from build123d import *

# Parameters (mm, degrees)
BOSS_EXTRUDE1_DEPTH     = 10
CUT_EXTRUDE1_DEPTH      = 26.734218465
CUT_EXTRUDE1_DEPTH_BACK = 26.734218465
SKETCH2_R               = 3.1
SKETCH3_R               = 2
CUT_EXTRUDE2_DEPTH      = 8.5


with BuildPart() as part:
    # Sketch1 → Boss-Extrude1 (new, symmetric)
    with BuildSketch(Plane.XY):
        with BuildLine():
            Line((-8, -21.5), (8, -21.5))
            ThreePointArc((8, -21.5), (9.414213562, -20.914213562), (10, -19.5))
            Line((10, -19.5), (10, -2))
            ThreePointArc((10, -2), (9.414213562, -0.585786438), (8, 0))
            Line((8, 0), (-8, 0))
            ThreePointArc((-8, 0), (-9.414213562, -0.585786438), (-10, -2))
            Line((-10, -2), (-10, -19.5))
            ThreePointArc((-10, -19.5), (-9.414213562, -20.914213562), (-8, -21.5))
        make_face()
    extrude(amount=BOSS_EXTRUDE1_DEPTH, both=True)

    # Sketch2 → Cut-Extrude1 (cut, two sides: drawn at the far end of the back side and taken through both)
    with BuildSketch(Plane(origin=(0, 0, 0), x_dir=(0, 0, -1), z_dir=(1, 0, 0)).offset(-CUT_EXTRUDE1_DEPTH_BACK)):
        with Locations((0, -9.5)):
            Circle(SKETCH2_R)
    extrude(amount=CUT_EXTRUDE1_DEPTH + CUT_EXTRUDE1_DEPTH_BACK, mode=Mode.SUBTRACT)

    # Sketch3 → Cut-Extrude2 (cut)
    with BuildSketch(Plane(origin=(0, -21.5, 0), x_dir=(1, 0, 0), z_dir=(0, 1, 0))):
        with Locations(Location((0, 0, 0), (0, 0, 270))):
            Circle(SKETCH3_R)
    extrude(amount=CUT_EXTRUDE2_DEPTH, mode=Mode.SUBTRACT)


solid = part.part
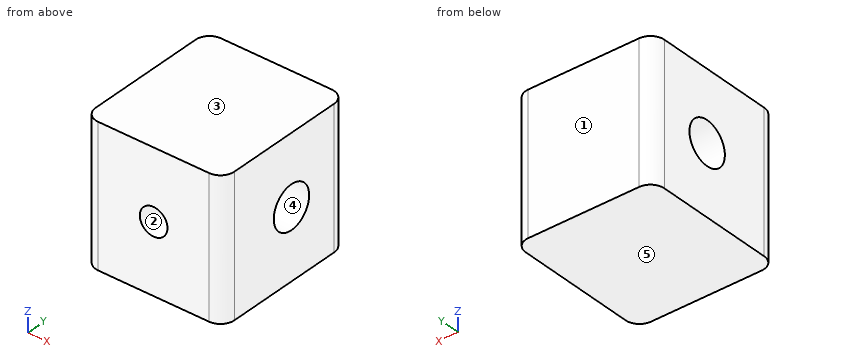
Read the model definition and answer for the solid it produces. Units are mm, in the model's axes. Face numbers are marked on the shaded views. A direction names the side the tool comes from. Round coordinates to 2 decimals unless told otherwise and drop trailing zeros. Loops run counter-clockwise (first coordinate to the right, second up) from the corner with the lowest first, then second, coordinate; pieces in that order, holes last.
Q1. This flat-tipped pin is pushed along its axis until it touches: pin 1 (3.5 mm diameter, centred on x = 0, z = 0, fed in from -Y). Where does it stop, or does it pass through?
Q2. Determine the mould class of the marked faces 3, 4 and 5 for opening direction Z: released by +Z, released by -Z, zero draft, split by the parting line, or undercut.
Q3. Consider probe 1 along Z at (x, y) = (0, -9.5); probe 2 along Y at (x, z) = (-7, 0); probe 3 along X at (y, z) = (-19.5, 0). Determine where each line is inside the solid, lowest interval first.
Q4. Section D-D on y = -18 is taken. Write down the section's boundary in (x, z), and give its area (3 significant figures).
Q5. Which of the six approach directions +Z, -Z, +X, -X, +Y, -Y give full straight-line access (tool end or side, diameter ignored) to the marked faces 1 and 2?
Q6. Section C-C on x = 0 is taken. Write down the section's boundary in (y, z), and give its area (3 significant figures).
Q7. Section A-A on y = -9.5 is taken. Write down the section's boundary in (x, z).
Q8. Section B-B on z = 0 is taken. Write down the section's boundary in (x, y).
Output:
1. pin 1: stops at y = -13
2. face 3: released by +Z
2. face 4: undercut
2. face 5: released by -Z
3. probe 1: z = -10 to -3.1, 3.1 to 10
3. probe 2: y = -21.5 to -12.6, -6.4 to 0
3. probe 3: x = -10 to -2, 2 to 10
4. outline: (-10, -10) - (10, -10) - (10, 10) - (-10, 10) - close; hole circle Ø4 at (0, 0)
4. area: 387 mm2
5. face 1: +Z, -Z, +X, -X, +Y
5. face 2: -Y
6. outline: (-21.5, -10) - (0, -10) - (0, 10) - (-21.5, 10) - (-21.5, 2) - (-13, 2) - (-13, -2) - (-21.5, -2) - close; hole circle Ø6.2 at (-9.5, 0)
6. area: 366 mm2
7. outline: (-10, -10) - (10, -10) - (10, -3.1) - (-10, -3.1) - close; (-10, 3.1) - (10, 3.1) - (10, 10) - (-10, 10) - close
8. outline: (-10, -19.5) arc R2 ccw to (-8, -21.5) - (-2, -21.5) - (-2, -13) - (2, -13) - (2, -21.5) - (8, -21.5) arc R2 ccw to (10, -19.5) - (10, -12.6) - (-10, -12.6) - close; (-10, -6.4) - (10, -6.4) - (10, -2) arc R2 ccw to (8, 0) - (-8, 0) arc R2 ccw to (-10, -2) - close
